Autodesk Inventor part; units mm, degrees
ref_plane "YZ Plane" through (0, 0, 0) normal (1, 0, 0) x (0, 1, 0)
ref_plane "XZ Plane" through (0, 0, 0) normal (0, 1, 0) x (-1, 0, 0)
ref_plane "XY Plane" through (0, 0, 0) normal (0, 0, 1) x (1, 0, 0)
sketch "Sketch1" plane through (0, 0, 0) normal (0, 0, 1) x (1, 0, 0)
  circle A0 centre (0, 0) radius 40
  dimension "d47" = 80
extrude "Extrusion1" add sketch "Sketch1" along normal blind 6
sketch "Sketch7" plane through (0, 0, 6) normal (0, 0, 1) x (1, 0, 0)
  circle A0 centre (0, 0) radius 40
  circle A1 centre (-36.828, 0) radius 1.5
  circle A2 centre (-26.0413, -26.0413) radius 1.5
  circle A3 centre (0, -36.828) radius 1.5
  circle A4 centre (26.0413, -26.0413) radius 1.5
  circle A5 centre (36.828, 0) radius 1.5
  circle A6 centre (26.0413, 26.0413) radius 1.5
  circle A7 centre (0, 36.828) radius 1.5
  circle A8 centre (-26.0413, 26.0413) radius 1.5
  dimension "d48" = 3
  dimension "d49" = 36.828
  dimension "d52" = 360
hole "Hole2" at (-26.0413, 26.0413, 6) at (0, 36.828, 6) at (26.0413, 26.0413, 6) at (36.828, 0, 6) at (26.0413, -26.0413, 6) at (0, -36.828, 6) at (-26.0413, -26.0413, 6) at (-36.828, 0, 6) direction (0, 0, -1) diameter 3.5052 end through all
sketch "Sketch8" plane through (0, 0, 6) normal (0, 0, 1) x (1, 0, 0)
  point P0 (0, 0)
  point P1 (0, 0)
hole "Hole3" at (0, 0, 6) direction (0, 0, -1) diameter 21.3 end through all
properties part number "Cover"
Verification items for the finished model (mm, model axes). Round coordinates to 2 decimals unless told otherwise and drop trailing zeros. Order: outer loops, then holes, each group sorted by start corner. A loop starts at its lowest first (then second) coordinate and runs counter-clockwise, first axis right, second up. Notation, with made-up numbers: (73, 35) -> (81, 35) arc R15 cw to (81, 52) -> close; hole circle Ø7 at (-1, 18.25). An arc over 180 degrees is marked (long way). Put each result on its own line as item: value. Start each with the question number.
(1) Depth check by flat-ended pin: pin 1 Ø5.5 at (x, y) = (0, 36.828) entering from +Z; pin 2 Ø1 at (y, z) = (6, 1.5) entering from -X; pin 3 Ø2 at (y, z) = (-16, 2) entering from +X; pin 4 Ø1 at (x, z) = (-15, 1) entering from -Y. Enter the tip coordinate at first touch or a pass-through.
(2) Section check A-A (y = 0). Enter the section's corners in (x, z).
(3) Draft check along Y on faces 1 (the face through (-8.67, 39.05, 2.96)), 2 (the face through (8, -8, 0)), 3 (the face through (-3.199, -10.158, 2.958)). Enter one of: +Y half, -Y half, draft (parallel to the pull), parting line (faces both ways), or undercut.
(4) Material ranges on line 1 along Y through (x, z) = (0, 1.8); line 2 along Y through (x, z) = (-1, 4.25); line 3 along X through (y, z) = (27, 2.9), recorded low to high.
(5) Section check C-C (y = -9). Enter the section's corners in (x, z).
(6) Section check D-D (z = 3.75). State how many separate pieces and enclosed holes the cut face has, then the cut area to 3 significant figures.
Completed:
1. pin 1: stops at z = 6
1. pin 2: stops at x = -39.62
1. pin 3: stops at x = 37.08
1. pin 4: stops at y = -37.28
2. outline: (-40, 0) -> (-38.58, 0) -> (-38.58, 6) -> (-40, 6) -> close; (-35.08, 0) -> (-10.65, 0) -> (-10.65, 6) -> (-35.08, 6) -> close; (10.65, 0) -> (35.08, 0) -> (35.08, 6) -> (10.65, 6) -> close; (38.58, 0) -> (40, 0) -> (40, 6) -> (38.58, 6) -> close
3. face 1: parting line
3. face 2: draft
3. face 3: undercut
4. line 1: y = -40 to -38.58, -35.08 to -10.65, 10.65 to 35.08, 38.58 to 40
4. line 2: y = -39.99 to -38.27, -35.39 to -10.6, 10.6 to 35.39, 38.27 to 39.99
4. line 3: x = -29.51 to -27.51, -24.57 to 24.57, 27.51 to 29.51
5. outline: (-38.97, 0) -> (-5.69, 0) -> (-5.69, 6) -> (-38.97, 6) -> close; (5.69, 0) -> (38.97, 0) -> (38.97, 6) -> (5.69, 6) -> close
6. separate pieces: 1
6. enclosed holes: 9
6. area: 4,590 mm2
